Work out the finished part from the listing and answer in its coordinate system (mm). Round coordinates to 2 decimals unless told otherwise and drop trailing zeros. Order: outer loops, then holes, each group sorted by start corner. A loop starts at its lowest first (then second) coordinate and runs counter-clockwise, first axis right, second up.
Autodesk Inventor part; units mm, degrees
ref_plane "YZ Plane" through (0, 0, 0) normal (1, 0, 0) x (0, 1, 0)
ref_plane "XZ Plane" through (0, 0, 0) normal (0, 1, 0) x (-1, 0, 0)
ref_plane "XY Plane" through (0, 0, 0) normal (0, 0, 1) x (1, 0, 0)
sketch "Sketch1" plane through (0, 0, 0) normal (0, 1, 0) x (-1, 0, 0)
  line L0 (-3.175, -3.175) -> (3.175, -3.175)
  line L1 (3.175, -3.175) -> (3.175, 3.175)
  line L2 (3.175, 3.175) -> (-3.175, 3.175)
  line L3 (-3.175, 3.175) -> (-3.175, -3.175)
  line L4 (-3.175, -3.175) -> (3.175, 3.175) construction
  line L5 (3.175, -3.175) -> (-3.175, 3.175) construction
  point P0 (0, 0)
  dimension "d0" = 6.35
  dimension "d1" = 6.35
extrude "Extrusion1" add sketch "Sketch1" along normal blind 76.2
fillet "Fillet1" radius 1.5875 4 edges at (3.175, 38.1, -3.175) (-3.175, 38.1, -3.175) (3.175, 38.1, 3.175) (-3.175, 38.1, 3.175)
fillet "Fillet2" radius 0.7937 16 edges at (3.175, 0, 0) (2.71, 0, -2.71) (0, 0, -3.175) (-2.71, 0, -2.71) (-3.175, 0, 0) (-2.71, 0, 2.71) (0, 0, 3.175) (2.71, 0, 2.71) (0, 76.2, 3.175) (-2.71, 76.2, 2.71) (-3.175, 76.2, 0) (-2.71, 76.2, -2.71) (0, 76.2, -3.175) (2.71, 76.2, -2.71) (3.175, 76.2, 0) (2.71, 76.2, 2.71)
properties part number "3inch" material "Stainless Steel"
Item 1: Given pin 1 (1 mm diameter, centred on x = 1, z = 1, fed in from -Y), flat-ended and moving along its own axis, determine where the tip first touches the part or whether it passes through.
Item 2: Find section A-A (y = 34.5). Write down the section's boundary in (x, z) (1 decimal).
Item 3: Find the intervals of material crossed by line 1 along X through (y, z) = (44, 1.75); line 2 along Y through (x, z) = (-0.75, 3), in increasing order.
Model answer:
1. pin 1: stops at y = 0
2. outline: (-3.2, -1.6) arc R1.6 ccw to (-1.6, -3.2) - (1.6, -3.2) arc R1.6 ccw to (3.2, -1.6) - (3.2, 1.6) arc R1.6 ccw to (1.6, 3.2) - (-1.6, 3.2) arc R1.6 ccw to (-3.2, 1.6) - close
3. line 1: x = -3.17 to 3.17
3. line 2: y = 0.3 to 75.9
